Design review of the part built by this model. Coordinates are the model's own, in mm. Coordinates: 2 decimals unless noted, no trailing zeros. Order: outer loops, then holes, each group sorted by start corner. A loop starts at its lowest first (then second) coordinate and runs counter-clockwise, first axis right, second up. Notation, with made-up numbers: (49, -6) - (70, -6) arc R11 cw to (70, 10) - close; hole circle Ø7 at (78.5, 46). An arc over 180 degrees is marked (long way). Write item = value, one per line. Start each with the question number.
```python
from build123d import *

# Parameters (mm, degrees)
CIRCLE023_R        = 2.2
EXTRUSION080_DEPTH = 24.9014
EXTRUSION079_DEPTH = 1.5


with BuildPart() as extrusion080:
    # Circle023 → Extrusion080 (new body)
    with BuildSketch(Plane(origin=(-317.078363, 162.03651, 0.266052), x_dir=(0, -1, 0), z_dir=(-1, 0, 0))):
        Circle(CIRCLE023_R)
    extrude(amount=-EXTRUSION080_DEPTH)


with BuildPart() as cut010012012:
    # Wire006 → Extrusion079 (new body)
    with BuildSketch(Plane(origin=(-317.078363, 158.399203, -1.833948), x_dir=(0, -1, 0), z_dir=(-1, 0, 0))):
        Polygon((0, 0), (-3.637307, -2.1), (-7.274613, 0), (-7.274613, 4.2), (-3.637307, 6.3), (0, 4.2), align=None)
    extrude(amount=-EXTRUSION079_DEPTH)

    # Cut010012012: cut Extrusion080
    add(extrusion080.part, mode=Mode.SUBTRACT)


solid = cut010012012.part
```
Item 1: Add section B-B on y = 160. Give the boundary of the cut face in (x, z).
Item 2: Add section C-C on x = -316. Give the boundary of the cut face in (y, z), plus the area to 3 significant figures.
Item 3: Add section A-A on z = 0.75. Give the boundary of the cut face in (x, y).
Item 4: Mouldability with a two-part tool opening along Y and no side actions: class faces 1 (the flat face through (-316.34, 160.19, -2.87)), 2 (the cylindrical face through (-316.34, 159.94, 0.93)), 3 (the flat face through (-317.078, 164, -2)) as +Y half, -Y half, draft (parallel to the pull), parting line (faces both ways), or undercut.
Item 5: Add section D-D on z = -2.25. Give the boundary of the cut face in (x, y).
Item 6: For line 1 (Y direction, x = -316.5, z = 0.25); line 2 (Y direction, x = -316.1, z = -1); line 3 (Z direction, x = -316.8, y = 164), list the stretches that pass through material, from the lowest coordinate up.
Worked out:
q1.outline = (-317.08, -2.76) - (-315.58, -2.76) - (-315.58, -0.57) - (-317.08, -0.57) - close; (-317.08, 1.1) - (-315.58, 1.1) - (-315.58, 3.29) - (-317.08, 3.29) - close
q2.outline = (158.4, -1.83) - (162.04, -3.93) - (165.67, -1.83) - (165.67, 2.37) - (162.04, 4.47) - (158.4, 2.37) - close; hole circle Ø4.4 at (162.04, 0.27)
q2.area = 30.6 mm2
q3.outline = (-317.08, 158.4) - (-315.58, 158.4) - (-315.58, 159.89) - (-317.08, 159.89) - close; (-317.08, 164.18) - (-315.58, 164.18) - (-315.58, 165.67) - (-317.08, 165.67) - close
q4.face_1 = -Y half
q4.face_2 = undercut
q4.face_3 = draft
q5.outline = (-317.08, 159.12) - (-315.58, 159.12) - (-315.58, 164.95) - (-317.08, 164.95) - close
q6.line_1 = 158.4 to 159.84, 164.24 to 165.67
q6.line_2 = 158.4 to 160.24, 163.84 to 165.67
q6.line_3 = -2.8 to -0.73, 1.26 to 3.33
